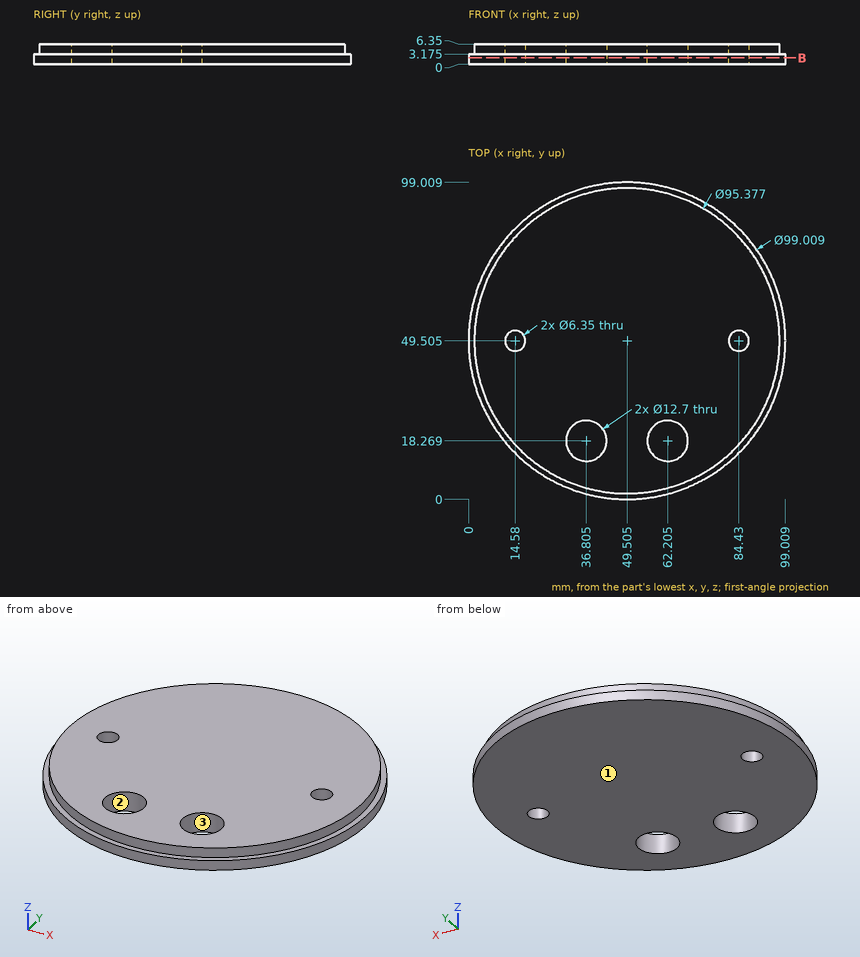
Can you work these out from the drawing? Everything is in mm from the part's minimum corner. Round coordinates to 2 decimals unless told otherwise and drop trailing zeros. Return JSON: item names as keys, results as strings. Group by question number.
1. If we section it at B-B, the plane z = 2: Count the separate pieces of the cut face and the enclosed holes in it, then the cut area to 3 significant figures.
2. I need wall thicknesses on line 1 (X direction, y = 15.5, z = 4.5); line 2 (X direction, y = 16, z = 4.75) (1 decimal); line 3 (Y direction, x = 39, z = 1.5). Which ranges of each line are inside material? Lowest first, please. Write a range as [from, to].
3. We'd pull the mould along Y, two halves only. Please class the marked faces 1, 2 and 3: released by +Y, released by -Y, zero draft, split by the parting line, or undercut.
4. Will these pins go through, and if not, where does the flat tip stop? pin 1 (3 mm diameter, centred on y = 46.5, z = 3, fed in from -X); pin 2 (8.5 mm diameter, centred on x = 84.43, y = 49.5, fed in from -Z); pin 3 (1.5 mm diameter, centred on y = 10, z = 2, fed in from +X).
Output values:
{
 "1": {"separate pieces": "1", "enclosed holes": "4", "area": "7,380 mm²"},
 "2": {"line 1": "[16.07, 31.09], [42.52, 56.49], [67.92, 82.94]", "line 2": "[15.6, 30.9], [42.7, 56.3], [68.1, 83.4]", "line 3": "[1.13, 12.31], [24.23, 97.88]"},
 "3": {"face 1": "zero draft", "face 2": "undercut", "face 3": "undercut"},
 "4": {"pin 1": "x = 0.02", "pin 2": "z = 0", "pin 3": "x = 80.31"}
}
